Answer from the drawing. Dimensions are ordinates in mm from the lowest x, y and z of the part. Round coordinates to 2 decimals unless told otherwise and drop trailing zeros. Loops run counter-clockwise (first coordinate to the right, second up) from the corner with the lowest first, then second, coordinate; pieces in that order, holes last.
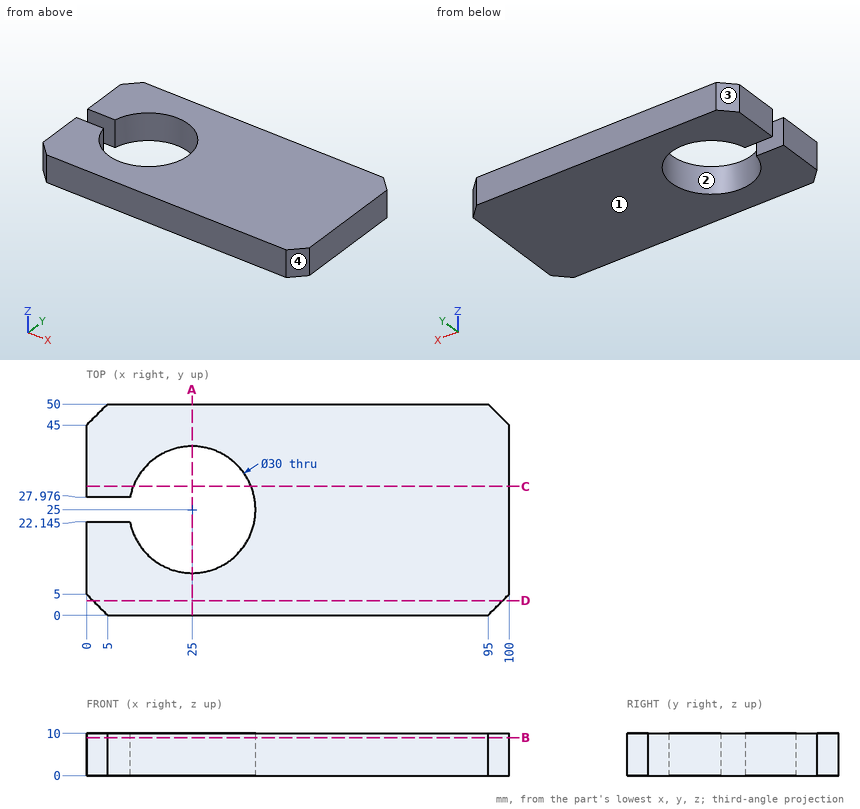
1. Consider probe 1 along Y at (x, z) = (25, 5); probe 2 along Y at (x, z) = (17, 7.5); probe 3 along X at (y, z) = (13, 4.25). Determine where each line is inside the solid, lowest interval first.
Answer key:
probe 1: y = 0 to 10, 40 to 50
probe 2: y = 0 to 12.31, 37.69 to 50
probe 3: x = 0 to 16, 34 to 100
2. Find section D-D (y = 3.5). Write down the section's boundary in (x, z), then the cut area to 3 significant figures.
Answer key:
outline: (1.5, 0) - (98.5, 0) - (98.5, 10) - (1.5, 10) - close
area: 970 mm2
3. Given pin 1 (3 mm diameter, centred on x = 5.5, z = 3, fed in from -Y), flat-ended and moving along its own axis, determine where the tip first touches the part or whether it passes through.
Answer key:
pin 1: stops at y = 0
4. Find section A-A (x = 25). Write down the section's boundary in (y, z).
Answer key:
outline: (0, 0) - (10, 0) - (10, 10) - (0, 10) - close; (40, 0) - (50, 0) - (50, 10) - (40, 10) - close
5. Find section B-B (z = 9). Write down the section's boundary in (x, y) (1 decimal).
Answer key:
outline: (0, 5) - (5, 0) - (95, 0) - (100, 5) - (100, 45) - (95, 50) - (5, 50) - (0, 45) - (0, 28) - (10.3, 28) arc R15 cw (long way) to (10.3, 22.1) - (0, 22.1) - close
6. Find section C-C (y = 30.5). Write down the section's boundary in (x, z) (1 decimal).
Answer key:
outline: (0, 0) - (11, 0) - (11, 10) - (0, 10) - close; (39, 0) - (100, 0) - (100, 10) - (39, 10) - close
7. Determine the mould class of the marked faces 1, 2, 3 and 4 for opening direction Y: +Y half, -Y half, draft (parallel to the pull), parting line (faces both ways), or undercut.
Answer key:
face 1: draft
face 2: undercut
face 3: +Y half
face 4: -Y half
